The listing builds one solid part. Answer for the finished solid, in the listing's coordinates (mm). Face numbers are marked on the shaded views. A direction names the side the tool comes from. Coordinates: 2 decimals unless noted, no trailing zeros. Write each loop counter-clockwise with the first axis right and the second up, starting at its lowest first coordinate (ties: lowest second). Pieces come first, ordered by that corner, then holes.
Autodesk Inventor part; units mm, degrees
ref_plane "YZ Plane" through (0, 0, 0) normal (1, 0, 0) x (0, 1, 0)
ref_plane "XZ Plane" through (0, 0, 0) normal (0, 1, 0) x (-1, 0, 0)
ref_plane "XY Plane" through (0, 0, 0) normal (0, 0, 1) x (1, 0, 0)
sketch "Sketch1" plane through (0, 0, 0) normal (0, 1, 0) x (-1, 0, 0)
  line L0 (0, 0) -> (0, -22.225)
  line L1 (0, -22.225) -> (15.875, -22.225)
  line L2 (15.875, -22.225) -> (15.875, 15.875)
  line L3 (15.875, 15.875) -> (-22.225, 15.875)
  line L4 (-22.225, 15.875) -> (-22.225, 0)
  line L5 (-22.225, 0) -> (0, 0)
  dimension "d0" = 15.875
  dimension "d1" = 38.1
extrude "Extrusion1" add sketch "Sketch1" against normal blind 15.875
sketch "Sketch3" plane through (0, 0, -22.225) normal (0, 0, -1) x (-1, 0, 0)
  line L0 (5.1145, -3.048) -> (10.7605, -3.048)
  line L1 (10.7605, -3.048) -> (13.5834, -7.9375)
  line L2 (13.5834, -7.9375) -> (10.7605, -12.827)
  line L3 (10.7605, -12.827) -> (5.1145, -12.827)
  line L4 (5.1145, -12.827) -> (2.2916, -7.9375)
  line L5 (2.2916, -7.9375) -> (5.1145, -3.048)
  line L6 (15.875, -15.875) -> (0, -15.875)
  line L7 (0, 0) -> (0, -15.875)
  point P0 (7.9375, -7.9375)
  dimension "d5" = 7.9375
  dimension "d6" = 7.9375
  dimension "d7" = 9.779
extrude "Extrusion2" cut sketch "Sketch3" against normal blind 31.75
sketch "Sketch4" plane through (22.225, 0, 15.875) normal (1, 0, 0) x (0, 0, -1)
  line L0 (13.5834, -7.9375) -> (10.7605, -12.827)
  line L1 (10.7605, -12.827) -> (5.1145, -12.827)
  line L2 (5.1145, -12.827) -> (2.2916, -7.9375)
  line L3 (2.2916, -7.9375) -> (5.1145, -3.048)
  line L4 (5.1145, -3.048) -> (10.7605, -3.048)
  line L5 (10.7605, -3.048) -> (13.5834, -7.9375)
  line L6 (0, 0) -> (15.875, 0)
  line L7 (15.875, 0) -> (15.875, -15.875)
  point P0 (7.9375, -7.9375)
  dimension "d10" = 9.779
  dimension "d11" = 7.9375
  dimension "d12" = 7.9375
extrude "Extrusion3" cut sketch "Sketch4" against normal blind 31.75
sketch "Sketch5" plane through (0, 0, 0) normal (0, 1, 0) x (1, 0, 0)
  line L0 (-15.875, 22.225) -> (-15.875, -15.875)
  line L1 (-15.875, -15.875) -> (22.225, -15.875)
  line L2 (0, 22.225) -> (-15.875, 22.225)
  line L3 (22.225, -15.875) -> (22.225, 0)
  point P0 (0, 0)
  point P1 (-7.9375, 4.826)
  point P2 (4.826, -7.9375)
  dimension "d15" = 7.9375
  dimension "d16" = 7.9375
  dimension "d17" = 17.399
  dimension "d18" = 17.399
hole "Hole1" at (-7.9375, 0, -4.826) at (4.826, 0, 7.9375) direction (0, -1, 0) diameter 5.1054 end through all
fillet "Fillet1" radius 3.175 6 edges at (-15.875, -7.9375, 15.875) (0, -7.9375, 0) (11.1125, 0, 0) (0, 0, -11.1125) (3.175, 0, 15.875) (-15.875, 0, -3.175)
fillet "Fillet2" radius 3.175 5 edges at (-14.9451, -15.875, 14.9451) (4.7625, -15.875, 15.875) (-15.875, -15.875, -4.7625) (12.7, -15.875, 0) (0, -15.875, -12.7)
equation "\"d0\" = pieceWidth"
equation "\"d1\" = pieceLength"
equation "\"d2\" = pieceWidth"
equation "\"d7\" = hex"
equation "\"d8\" = depthOfHexCut"
equation "\"d10\" = hex"
equation "\"d13\" = depthOfHexCut"
equation "\"pieceWidth\" = 15.875"
equation "\"pieceLength\" = 38.1"
equation "\"depthOfInsert\" = 25.4"
equation "\"printingError\" = 0.254"
equation "\"depthForHexBracket\" = 17.399"
properties part number "3_8_angleJoint"
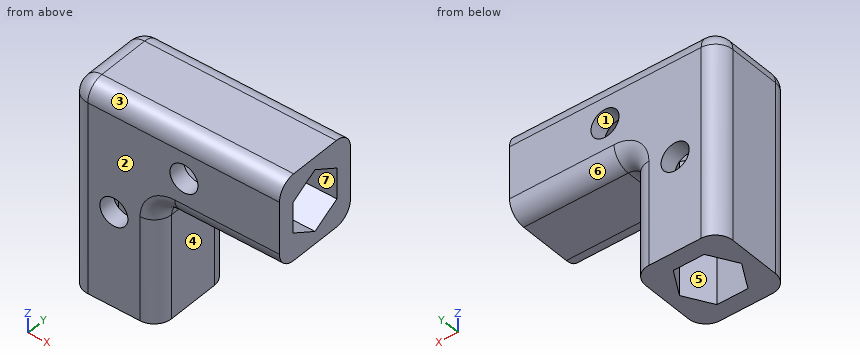
1. Find the intervals of material crossed by L1, parallel to Y at x = 12, z = 11 (3 decimals); L2, parallel to Y at x = -2.5, z = 3.5 (3 decimals); L3, parallel to X at y = -6, z = -18.5 (3 decimals), in increasing order.
Results found:
L1: y = -15.875 to -12.412, -3.463 to 0
L2: y = -15.875 to -10.031, -5.844 to 0
L3: x = -15.875 to -12.465, -3.41 to 0
2. Section C-C on y = -11.5 is taken. Give the vertices of the cut face in (x, z) (3 decimals).
Results found:
outline: (-15.875, -22.225) - (-11.527, -22.225) - (-11.527, 9.525) - (-9.525, 9.525) - (-9.525, 11.527) - (22.225, 11.527) - (22.225, 15.875) - (-12.7, 15.875) arc R3.175 ccw to (-15.875, 12.7) - close; (-4.348, -22.225) - (0, -22.225) - (0, -3.175) arc R3.175 cw to (3.175, 0) - (22.225, 0) - (22.225, 4.348) - (-4.348, 4.348) - close
3. For a pull along Z with two mould halves and no side action, classify the marked faces 1, 2 and 3 as pulls with the +Z half, pulls with the -Z half, needs draft (parallel to the pull), parting line crosses it, or undercut.
Results found:
face 1: undercut
face 2: needs draft
face 3: pulls with the +Z half
4. A tool of negligible diameter and unlimited length cuts with its end or side. For the marked faces 4, 5, 6 and 7, from which of +Z, -Z, +X, -X, +Y, -Y can it reach the whole face along a straight path? Write none if from no direction.
Results found:
face 4: -Z, +X, +Y, -Y
face 5: -Z
face 6: -Z, +X, +Y
face 7: none
5. Flat-ended cylindrical pins translate along their axes: P1, Ø2, axis at x = 6.5, y = -7, coming from the -Z side; P2, Ø2, axis at x = 17, y = -1.5, coming from the -Z side; P3, Ø1.2, axis at y = -9.5, z = 11, coming from the +X side (3 decimals). Find the tip coordinate at first contact, or state that the pin passes through.
Results found:
P1: stops at z = 0
P2: stops at z = 0.07
P3: stops at x = -9.525
